Read the model definition and answer for the solid it produces. Units are mm, in the model's axes. A direction names the side the tool comes from. Coordinates: 2 decimals unless noted, no trailing zeros. Write each loop counter-clockwise with the first axis right and the second up, starting at its lowest first coordinate (ties: lowest second). Pieces come first, ordered by that corner, then holes. Notation, with made-up numbers: (38, 38) -> (85, 38) arc R16 cw to (85, 62) -> close; hole circle Ø1 at (69.25, 26). An arc over 180 degrees is marked (long way). One line per item, written item: value. Start each with the question number.
1. Consider line 1 along X through (y, z) = (-2.5, 5); line 2 along X through (y, z) = (-2.1, 5); line 3 along X through (y, z) = (-5.5, 1.75). Determine where each line is inside the solid, lowest interval first.
2. Find section D-D, the plane x = 0. Write down the section's boundary in (y, z), and give its area (3 significant figures).
3. Find section C-C, the plane y = -16.5. Write down the section's boundary in (x, z).
4. Given P1, Ø2, axis at x = -27, z = 5, coming from the +Y side; P2, Ø1, axis at x = 7.5, z = 8, coming from the +Y side; P3, Ø3, axis at x = 9, z = 2, coming from the -Y side; P4, Ø5.5, axis at x = 27, z = 5, coming from the -Y side, each flat-ended and moving along its own axis, determine where each tip first touches the part or whether it passes through.
5. For faces 5 (the flat face through (25, -6.3, 5)), 6 (the flat face through (-25, -0.3, 5)), 7 (the flat face through (-29, -6.3, 5)), determine the directions among +Z, -Z, +X, -X, +Y, -Y from which every point of the face is accessible in a straight line to the end or side of a thin tool.
6. For a pull along Z with two mould halves and no side action, classify faces 1 (the flat face through (-2.5, -17.5, 10)), 2 (the cylindrical face through (-28.686, -3.342, 5.221)), 3 (the flat face through (-32, -3, 5)), 4 (the flat face through (-2.5, -17.5, 0)) as pulls with the +Z half, pulls with the -Z half, needs draft (parallel to the pull), parting line crosses it, or undercut.
7. Find section B-B, the plane x = 27. Write down the section's boundary in (y, z), and give its area (3 significant figures).
```python
from build123d import *

# Parameters (mm, degrees)
F_01_REAR_SEMICIRCULAR_CAP_AND_BOLT_EARS_DEPTH = 10
F_02_START                                     = -0.2
S02_MATING_MOTOR_CAN_R                         = 17.4
F_02_MATING_MOTOR_CAN_DEPTH                    = 10.4
F_03_START                                     = -6.5
S03_TWO_M3_CLAMP_SCREWS_R                      = 1.7
F_03_TWO_M3_CLAMP_SCREWS_DEPTH                 = 6.7


with BuildPart() as part:
    # S01 - Rear semicircular cap and bolt ears → 01 - Rear semicircular cap and bolt ears (new body)
    with BuildSketch(Plane.XY):
        with BuildLine():
            Line((-32, -0.3), (-32, -6.3))
            Line((-32, -6.3), (-22.1, -6.3))
            ThreePointArc((-22.1, -6.3), (0, -23), (22.1, -6.3))
            Line((22.1, -6.3), (32, -6.3))
            Line((32, -6.3), (32, -0.3))
            Line((32, -0.3), (-32, -0.3))
        make_face()
    extrude(amount=F_01_REAR_SEMICIRCULAR_CAP_AND_BOLT_EARS_DEPTH)

    # S02 - Mating motor can → 02 - Mating motor can (cut)
    with BuildSketch(Plane.XY.offset(F_02_START)):
        Circle(S02_MATING_MOTOR_CAN_R)
    extrude(amount=F_02_MATING_MOTOR_CAN_DEPTH, mode=Mode.SUBTRACT)

    # S03 - Two M3 clamp screws → 03 - Two M3 clamp screws (cut)
    with BuildSketch(Plane(origin=(0, 0, 0), x_dir=(1, 0, 0), z_dir=(0, 1, 0)).offset(F_03_START)):
        with Locations(Location((-27, -5, 0), (0, 0, 90))):
            Circle(S03_TWO_M3_CLAMP_SCREWS_R)
        with Locations(Location((27, -5, 0), (0, 0, 90))):
            Circle(S03_TWO_M3_CLAMP_SCREWS_R)
    extrude(amount=F_03_TWO_M3_CLAMP_SCREWS_DEPTH, mode=Mode.SUBTRACT)


solid = part.part
```
Answer block:
1. line 1: x = -32 to -28.7, -25.3 to -17.22, 17.22 to 25.3, 28.7 to 32
1. line 2: x = -32 to -28.7, -25.3 to -17.27, 17.27 to 25.3, 28.7 to 32
1. line 3: x = -32 to -16.51, 16.51 to 32
2. outline: (-23, 0) -> (-17.4, 0) -> (-17.4, 10) -> (-23, 10) -> close
2. area: 56.0 mm2
3. outline: (-16.01, 0) -> (-5.52, 0) -> (-5.52, 10) -> (-16.01, 10) -> close; (5.52, 0) -> (16.01, 0) -> (16.01, 10) -> (5.52, 10) -> close
4. P1: passes through
4. P2: stops at y = -15.45
4. P3: stops at y = -21.74
4. P4: stops at y = -6.3
5. face 5: +Z, -Z, +X, -Y
5. face 6: +Z, -Z, +X, -X, +Y
5. face 7: +Z, -Z, -X, -Y
6. face 1: pulls with the +Z half
6. face 2: undercut
6. face 3: needs draft
6. face 4: pulls with the -Z half
7. outline: (-6.3, 0) -> (-0.3, 0) -> (-0.3, 3.3) -> (-6.3, 3.3) -> close; (-6.3, 6.7) -> (-0.3, 6.7) -> (-0.3, 10) -> (-6.3, 10) -> close
7. area: 39.6 mm2
